CAD build for the part. Positions are in the model's coordinates, mm. Round coordinates to 2 decimals unless told otherwise and drop trailing zeros. Order: outer loops, then holes, each group sorted by start corner. A loop starts at its lowest first (then second) coordinate and runs counter-clockwise, first axis right, second up. Notation, with made-up numbers: M -30.5,84.5 L 14.5,84.5 A16 cw 14.5,109.5 Z; hole C 72,29.5 d2. An arc over 180 degrees is marked long. Answer as a JSON object with one key per item and string values.
```python
from build123d import *

# Parameters (mm, degrees)
ESQUISSE1_R        = 4.5
ESQUISSE1_R_2      = 4
BOSS_EXTRU_1_DEPTH = 12
CHANFREIN1_SIZE    = 3


with BuildPart() as part:
    # Esquisse1 → Boss.-Extru.1 (new body)
    with BuildSketch(Plane(origin=(0, 0, 0), x_dir=(1, 0, 0), z_dir=(0, 1, 0))):
        Polygon((0, -75), (64.951905284, -37.5), (64.951905284, 37.5), (0, 75), (-64.951905284, 37.5), (-64.951905284, -37.5), align=None)
        with Locations(Location((0, 0, 0), (0, 0, 270))):
            Circle(ESQUISSE1_R, mode=Mode.SUBTRACT)
        with Locations(Location((0, 20, 0), (0, 0, 270))):
            Circle(ESQUISSE1_R, mode=Mode.SUBTRACT)
        with Locations(Location((0, 35, 0), (0, 0, 270))):
            Circle(ESQUISSE1_R, mode=Mode.SUBTRACT)
        with Locations(Location((0, 50, 0), (0, 0, 270))):
            Circle(ESQUISSE1_R, mode=Mode.SUBTRACT)
        with Locations(Location((0, 65, 0), (0, 0, 270))):
            Circle(ESQUISSE1_R, mode=Mode.SUBTRACT)
        with Locations(Location((17.320508076, 10, 0), (0, 0, 270))):
            Circle(ESQUISSE1_R, mode=Mode.SUBTRACT)
        with Locations(Location((30.310889132, 17.5, 0), (0, 0, 270))):
            Circle(ESQUISSE1_R, mode=Mode.SUBTRACT)
        with Locations(Location((43.301270189, 25, 0), (0, 0, 270))):
            Circle(ESQUISSE1_R, mode=Mode.SUBTRACT)
        with Locations(Location((56.291651246, 32.5, 0), (0, 0, 270))):
            Circle(ESQUISSE1_R, mode=Mode.SUBTRACT)
        with Locations(Location((17.320508076, -10, 0), (0, 0, 270))):
            Circle(ESQUISSE1_R, mode=Mode.SUBTRACT)
        with Locations(Location((30.310889132, -17.5, 0), (0, 0, 270))):
            Circle(ESQUISSE1_R, mode=Mode.SUBTRACT)
        with Locations(Location((43.301270189, -25, 0), (0, 0, 270))):
            Circle(ESQUISSE1_R, mode=Mode.SUBTRACT)
        with Locations(Location((56.291651246, -32.5, 0), (0, 0, 270))):
            Circle(ESQUISSE1_R, mode=Mode.SUBTRACT)
        with Locations(Location((0, -20, 0), (0, 0, 270))):
            Circle(ESQUISSE1_R, mode=Mode.SUBTRACT)
        with Locations(Location((0, -35, 0), (0, 0, 270))):
            Circle(ESQUISSE1_R, mode=Mode.SUBTRACT)
        with Locations(Location((0, -50, 0), (0, 0, 270))):
            Circle(ESQUISSE1_R, mode=Mode.SUBTRACT)
        with Locations(Location((0, -65, 0), (0, 0, 270))):
            Circle(ESQUISSE1_R, mode=Mode.SUBTRACT)
        with Locations(Location((-17.320508076, -10, 0), (0, 0, 270))):
            Circle(ESQUISSE1_R, mode=Mode.SUBTRACT)
        with Locations(Location((-30.310889132, -17.5, 0), (0, 0, 270))):
            Circle(ESQUISSE1_R, mode=Mode.SUBTRACT)
        with Locations(Location((-43.301270189, -25, 0), (0, 0, 270))):
            Circle(ESQUISSE1_R, mode=Mode.SUBTRACT)
        with Locations(Location((-56.291651246, -32.5, 0), (0, 0, 270))):
            Circle(ESQUISSE1_R, mode=Mode.SUBTRACT)
        with Locations(Location((-17.320508076, 10, 0), (0, 0, 270))):
            Circle(ESQUISSE1_R, mode=Mode.SUBTRACT)
        with Locations(Location((-30.310889132, 17.5, 0), (0, 0, 270))):
            Circle(ESQUISSE1_R, mode=Mode.SUBTRACT)
        with Locations(Location((-43.301270189, 25, 0), (0, 0, 270))):
            Circle(ESQUISSE1_R, mode=Mode.SUBTRACT)
        with Locations(Location((-56.291651246, 32.5, 0), (0, 0, 270))):
            Circle(ESQUISSE1_R, mode=Mode.SUBTRACT)
        with Locations(Location((17.320508076, 0, 0), (0, 0, 270))):
            Circle(ESQUISSE1_R_2, mode=Mode.SUBTRACT)
        with Locations(Location((30.310889132, 0, 0), (0, 0, 270))):
            Circle(ESQUISSE1_R_2, mode=Mode.SUBTRACT)
        with Locations(Location((43.301270189, 0, 0), (0, 0, 270))):
            Circle(ESQUISSE1_R_2, mode=Mode.SUBTRACT)
        with Locations(Location((56.291651246, 0, 0), (0, 0, 270))):
            Circle(ESQUISSE1_R_2, mode=Mode.SUBTRACT)
        with Locations(Location((8.660254038, -15, 0), (0, 0, 270))):
            Circle(ESQUISSE1_R_2, mode=Mode.SUBTRACT)
        with Locations(Location((15.155444566, -26.25, 0), (0, 0, 270))):
            Circle(ESQUISSE1_R_2, mode=Mode.SUBTRACT)
        with Locations(Location((21.650635095, -37.5, 0), (0, 0, 270))):
            Circle(ESQUISSE1_R_2, mode=Mode.SUBTRACT)
        with Locations(Location((28.145825623, -48.75, 0), (0, 0, 270))):
            Circle(ESQUISSE1_R_2, mode=Mode.SUBTRACT)
        with Locations(Location((-8.660254038, -15, 0), (0, 0, 270))):
            Circle(ESQUISSE1_R_2, mode=Mode.SUBTRACT)
        with Locations(Location((-15.155444566, -26.25, 0), (0, 0, 270))):
            Circle(ESQUISSE1_R_2, mode=Mode.SUBTRACT)
        with Locations(Location((-21.650635095, -37.5, 0), (0, 0, 270))):
            Circle(ESQUISSE1_R_2, mode=Mode.SUBTRACT)
        with Locations(Location((-28.145825623, -48.75, 0), (0, 0, 270))):
            Circle(ESQUISSE1_R_2, mode=Mode.SUBTRACT)
        with Locations(Location((-17.320508076, 0, 0), (0, 0, 270))):
            Circle(ESQUISSE1_R_2, mode=Mode.SUBTRACT)
        with Locations(Location((-30.310889132, 0, 0), (0, 0, 270))):
            Circle(ESQUISSE1_R_2, mode=Mode.SUBTRACT)
        with Locations(Location((-43.301270189, 0, 0), (0, 0, 270))):
            Circle(ESQUISSE1_R_2, mode=Mode.SUBTRACT)
        with Locations(Location((-56.291651246, 0, 0), (0, 0, 270))):
            Circle(ESQUISSE1_R_2, mode=Mode.SUBTRACT)
        with Locations(Location((-8.660254038, 15, 0), (0, 0, 270))):
            Circle(ESQUISSE1_R_2, mode=Mode.SUBTRACT)
        with Locations(Location((-15.155444566, 26.25, 0), (0, 0, 270))):
            Circle(ESQUISSE1_R_2, mode=Mode.SUBTRACT)
        with Locations(Location((-21.650635095, 37.5, 0), (0, 0, 270))):
            Circle(ESQUISSE1_R_2, mode=Mode.SUBTRACT)
        with Locations(Location((-28.145825623, 48.75, 0), (0, 0, 270))):
            Circle(ESQUISSE1_R_2, mode=Mode.SUBTRACT)
        with Locations(Location((8.660254038, 15, 0), (0, 0, 270))):
            Circle(ESQUISSE1_R_2, mode=Mode.SUBTRACT)
        with Locations(Location((15.155444566, 26.25, 0), (0, 0, 270))):
            Circle(ESQUISSE1_R_2, mode=Mode.SUBTRACT)
        with Locations(Location((21.650635095, 37.5, 0), (0, 0, 270))):
            Circle(ESQUISSE1_R_2, mode=Mode.SUBTRACT)
        with Locations(Location((28.145825623, 48.75, 0), (0, 0, 270))):
            Circle(ESQUISSE1_R_2, mode=Mode.SUBTRACT)
    extrude(amount=BOSS_EXTRU_1_DEPTH)

    # Chanfrein1
    chanfrein1_edges = [part.edges().sort_by_distance(p)[0] for p in [
        (32.475952642, 12, 56.25),
        (64.951905284, 12, 0),
        (32.475952642, 12, -56.25),
        (-32.475952642, 12, -56.25),
        (-64.951905284, 12, 0),
        (-32.475952642, 12, 56.25),
    ]]
    chamfer(chanfrein1_edges, length=CHANFREIN1_SIZE)


solid = part.part
```
Item 1: Saw through at A-A on z = -48.75. List the corners of the cut face in (x, y), and give its area (3 significant figures).
Worked answers:
{"outline": "M -45.47,0 L -32.15,0 L -32.15,12 L -39.47,12 L -45.47,9 Z; M -24.15,0 L -4.32,0 L -4.32,12 L -24.15,12 Z; M 4.32,0 L 24.15,0 L 24.15,12 L 4.32,12 Z; M 32.15,0 L 45.47,0 L 45.47,9 L 39.47,12 L 32.15,12 Z", "area": "777 mm2"}
Item 2: Drop flat-ended pins along their axis: pin 1 Ø2 at (x, y) = (-8.5, 8) entering from -Z; pin 2 Ø1 at (y, z) = (6.5, -56.5) entering from -X; pin 3 Ø5.5 at (x, z) = (56.29, -32.5) entering from +Y; pin 4 Ø1.5 at (x, y) = (12.5, 2) entering from +Z. Give the stop position or say it passes through.
Worked answers:
{"pin 1": "stops at z = -70.67", "pin 2": "stops at x = -32.91", "pin 3": "passes through", "pin 4": "stops at z = 68.22"}
Item 3: Saw through at B-B on y = 5.25. State how many separate pieces and enclosed holes the cut face has, and give its area (3 significant figures).
Worked answers:
{"separate pieces": "1", "enclosed holes": "49", "area": "11,800 mm2"}
Item 4: Wall check: line 1 along Z through (x, y) = (42.5, 5.75); line 2 along X through (y, z) = (4.75, -23); line 3 along Z through (x, y) = (-20.5, 7). Give the ranges that are in metal, low to high. Write a range as [from, to].
Worked answers:
{"line 1": "z = [-50.46, -29.43], [-20.57, -3.92], [3.92, 20.57], [29.43, 50.46]", "line 2": "x = [-64.95, -47.33], [-39.27, -17.49], [-12.82, -3.35], [3.35, 12.82], [17.49, 39.27], [47.33, 64.95]", "line 3": "z = [-63.16, -41.33], [-33.67, -13.18], [-6.82, -2.43], [2.43, 6.82], [13.18, 33.67], [41.33, 63.16]"}
Item 5: Two-plate mould, pull along Z, no slides. Class faces 1 (the cylindrical face through (11.36, 5.92, 12.05)), 2 (the flat face through (-32.93, 4.44, 55.99)), 3 (the flat face through (32.93, 4.44, -55.99)): released by +Z, released by -Z, zero draft, split by the parting line, or undercut.
Worked answers:
{"face 1": "undercut", "face 2": "released by +Z", "face 3": "released by -Z"}
